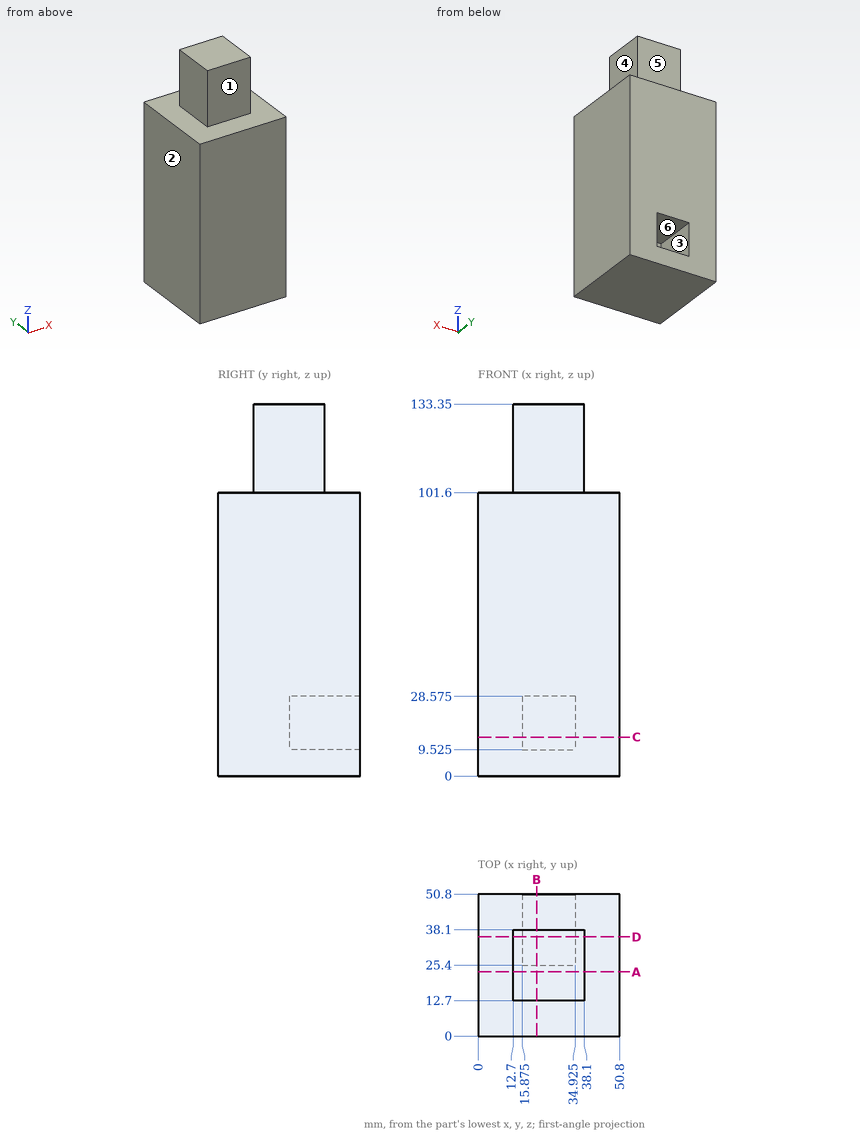
Study the drawing (mm; zero at the part's minimum x, y, z) and answer. A direction names the side the tool comes from. Give positions to 0.01 mm unless a question says otherwise; leave off trailing zeros. Write each loop counter-clockwise with the first axis right and the second up, starting at its lowest first coordinate (ties: lowest second). Pieces come first, ordered by that corner, then holes. Notation, with made-up numbers: (-37, 43) - (-20, 43) arc R18 ccw to (-20, 51) - close; hole circle Ø8 at (-28.75, 56.25). An arc over 180 degrees is marked (long way). Use a Markdown table: item, result.
1. Section D-D on y = 35.5 is taken. Write down the section's boundary in (x, z) (3 decimals).
Values follow:
| item | result |
|---|---|
| outline | (0, 0) - (50.8, 0) - (50.8, 101.6) - (38.1, 101.6) - (38.1, 133.35) - (12.7, 133.35) - (12.7, 101.6) - (0, 101.6) - close; hole (15.875, 9.525) - (34.925, 9.525) - (34.925, 28.575) - (15.875, 28.575) - close |
2. Section C-C on z = 14 is taken. Write down the section's boundary in (x, y) (3 decimals).
Values follow:
| item | result |
|---|---|
| outline | (0, 0) - (50.8, 0) - (50.8, 50.8) - (34.925, 50.8) - (34.925, 25.4) - (15.875, 25.4) - (15.875, 50.8) - (0, 50.8) - close |
3. A tool of negligible diameter and unlimited length cuts with its end or side. For the marked faces 4, 5 and 6, from which of +Z, -Z, +X, -X, +Y, -Y can it reach the whole face along a straight path? Write none if from no direction.
Values follow:
| item | result |
|---|---|
| face 4 | +Z, +X, +Y, -Y |
| face 5 | +Z, +X, -X, +Y |
| face 6 | +Y |
4. Section A-A on y = 23 is taken. Write down the section's boundary in (x, z).
Values follow:
| item | result |
|---|---|
| outline | (0, 0) - (50.8, 0) - (50.8, 101.6) - (38.1, 101.6) - (38.1, 133.35) - (12.7, 133.35) - (12.7, 101.6) - (0, 101.6) - close |
5. Find the intervals of material crossed by probe 1 along X at (y, z) = (44, 22.5) (3 decimals); probe 2 along Z at (x, y) = (31, 38.5) (3 decimals); probe 3 along Z at (x, y) = (47.5, 28), in increasing order. Write a range as from..to.
Values follow:
| item | result |
|---|---|
| probe 1 | x = 0..15.875, 34.925..50.8 |
| probe 2 | z = 0..9.525, 28.575..101.6 |
| probe 3 | z = 0..101.6 |
6. For a pull along X with two mould halves and no side action, classify the marked faces 1, 2 and 3 as released by +X, released by -X, zero draft, split by the parting line, or undercut.
Values follow:
| item | result |
|---|---|
| face 1 | zero draft |
| face 2 | released by -X |
| face 3 | undercut |
7. Each of these flat-tipped pins is pushed along its axis until it touches: P1, Ø1, axis at y = 25.5, z = 27, coming from the -X side; P2, Ø20.5, axis at x = 26.5, z = 120.5, coming from the +Y side; P3, Ø1.5, axis at y = 18, z = 104, coming from the +X side; P4, Ø12, axis at x = 5.5, z = 114.5, coming from the -Y side. Where does it stop, or does it pass through?
Values follow:
| item | result |
|---|---|
| P1 | stops at x = 0 |
| P2 | stops at y = 38.1 |
| P3 | stops at x = 38.1 |
| P4 | passes through |
8. Section B-B on x = 21 is taken. Write down the section's boundary in (y, z) (3 decimals).
Values follow:
| item | result |
|---|---|
| outline | (0, 0) - (50.8, 0) - (50.8, 9.525) - (25.4, 9.525) - (25.4, 28.575) - (50.8, 28.575) - (50.8, 101.6) - (38.1, 101.6) - (38.1, 133.35) - (12.7, 133.35) - (12.7, 101.6) - (0, 101.6) - close |
